Verification items for the finished model (mm, model axes). A direction names the side the tool comes from. Coordinates: 2 decimals unless noted, no trailing zeros. Loops run counter-clockwise (first coordinate to the right, second up) from the corner with the lowest first, then second, coordinate; pieces in that order, holes last. Notation, with made-up numbers: (-37, 73.5) - (13, 73.5) arc R28 cw to (13, 97.5) - close; hole circle Ø9 at (-19.5, -0.75). An arc over 180 degrees is marked (long way). One line per item, written item: value. Start each with the question number.
(1) Set-up check for faces 1 (the face through (-22.05, 5, 0)), 2 (the face through (-0.533, 3.491, 25.044)), 3 (the face through (15.799, 5.266, -11.984)): record each of +Z, -Z, +X, -X, +Y, -Y from which the full face is reachable in a straight line by a thin tool's end or side.
(2) Section check B-B (y = 3.25). Count the separate pieces of the cut face and the enclosed holes in it, plus the area to 3 significant figures.
(3) Gauge pin test, flat ends, axial feed: P1, Ø2, axis at y = 5.5, z = 0.5, coming from the +X side; P2, Ø0.8, axis at y = 3.5, z = 0.5, coming from the -X side; P3, Ø5, axis at x = 22, y = 5.5, coming from the +Z side; P4, Ø23.5, axis at x = 0, z = 0, coming from the -Y side. Record the tip position at first contact, or that the pin passes through.
(4) Draft check along Z on faces 4 (the face through (0.636, 10.258, -29.686)), 5 (the face through (24, 6, 1.25)), 6 (the face through (2, 6.4, 26)), 7 (the face through (7.91, 8.174, 10.316)). Enter one of: +Z half, -Z half, draft (parallel to the pull), parting line (faces both ways), or undercut.
(5) Thickness scan on probe 1 along X at (y, z) = (2, -0.5); probe 2 along Z at (x, y) = (18, 5.5); probe 3 along X at (y, z) = (6, 10). Record the ranges inside material, lowest first. Write a range as [from, to].
(6) Section check A-A (z = 0). Record the boundary of the cut face in (x, y) (3 decimals), plus the area to 3 significant figures.
```python
from build123d import *

# Parameters (mm, degrees)
SKETCH2_R               = 2.5
CUT_EXTRUDE1_DEPTH      = 44.751171413
SKETCH3_W               = 8
SKETCH3_H               = 2.5
CUT_EXTRUDE_THIN1_DEPTH = 44.751171413
CHAMFER1_SIZE           = 0.5


with BuildPart() as part:
    # Sketch1 → Revolve1 (revolve)
    with BuildSketch(Plane.XY, mode=Mode.PRIVATE) as revolve1_sk:
        Polygon((-15.975, 0), (-25.05, 0), (-25.05, 6.4), (-30.05, 6.4), (-30.05, 10.4), (-13, 10.4), (-13, 6.496321403), (-15.975, 4), align=None)
    revolve(revolve1_sk.sketch.rotate(Axis((0, 0, 0), (0, 1, 0)), 270), axis=Axis((0, 0, 0), (0, 1, 0)))

    # Sketch2 → Cut-Extrude1 (cut, through all)
    with BuildSketch(Plane(origin=(0, 10.4, 0), x_dir=(1, 0, 0), z_dir=(0, 1, 0))):
        with Locations(Location((0, 20, 0), (0, 0, 270))):
            Circle(SKETCH2_R)
        with Locations(Location((17.320508076, 10, 0), (0, 0, 270))):
            Circle(SKETCH2_R)
        with Locations(Location((17.320508076, -10, 0), (0, 0, 270))):
            Circle(SKETCH2_R)
        with Locations(Location((0, -20, 0), (0, 0, 270))):
            Circle(SKETCH2_R)
        with Locations(Location((-17.320508076, -10, 0), (0, 0, 270))):
            Circle(SKETCH2_R)
        with Locations(Location((-17.320508076, 10, 0), (0, 0, 270))):
            Circle(SKETCH2_R)
    extrude(amount=-CUT_EXTRUDE1_DEPTH, mode=Mode.SUBTRACT)

    # Sketch3 → Cut-Extrude-Thin1 (cut, through all)
    with BuildSketch(Plane(origin=(0, 10.4, 0), x_dir=(1, 0, 0), z_dir=(0, 1, 0))):
        with Locations((-26.05, 0)):
            Rectangle(SKETCH3_W, SKETCH3_H)
        with Locations((26.05, 0)):
            Rectangle(SKETCH3_W, SKETCH3_H)
    extrude(amount=-CUT_EXTRUDE_THIN1_DEPTH, mode=Mode.SUBTRACT)

    # Chamfer1
    chamfer1_edges = [part.edges().sort_by_distance(p)[0] for p in [
        (0, 0, 15.975),
        (0, 0, -22.5),
        (0, 10.4, -22.5),
        (-17.320508076, 0, -12.5),
        (-17.320508076, 10.4, -12.5),
        (-17.320508076, 0, 7.5),
        (-17.320508076, 10.4, 7.5),
        (0, 0, 17.5),
        (0, 10.4, 17.5),
        (17.320508076, 0, 7.5),
        (17.320508076, 10.4, 7.5),
        (17.320508076, 0, -12.5),
        (17.320508076, 10.4, -12.5),
        (0, 10.4, 30.05),
        (0, 10.4, -30.05),
        (26.036995204, 10.4, 1.25),
        (26.036995204, 10.4, -1.25),
        (-26.036995204, 10.4, -1.25),
        (-26.036995204, 10.4, 1.25),
        (0, 6.4, 30.05),
        (0, 6.4, -30.05),
        (0, 0, 25.05),
        (0, 0, -25.05),
        (-23.534396468, 0, -1.25),
        (-22.05, 0, 0),
        (-23.534396468, 0, 1.25),
        (-22.05, 10.4, 0),
        (0, 10.4, 13),
        (23.534396468, 0, 1.25),
        (22.05, 0, 0),
        (23.534396468, 0, -1.25),
        (22.05, 10.4, 0),
    ]]
    chamfer(chamfer1_edges, length=CHAMFER1_SIZE)


solid = part.part
```
Responses:
1. face 1: -X, +Y, -Y
1. face 2: +Z, -Y
1. face 3: +Y, -Y
2. separate pieces: 1
2. enclosed holes: 7
2. area: 1,040 mm²
3. P1: stops at x = 25.02
3. P2: stops at x = -22.05
3. P3: stops at z = 22.49
3. P4: passes through
4. face 4: -Z half
4. face 5: undercut
4. face 6: draft
4. face 7: undercut
5. probe 1: x = [-22.05, -15.97], [15.97, 22.05]
5. probe 2: z = [-17.42, -12.41], [-7.59, 7.59], [12.41, 17.42]
5. probe 3: x = [-22.97, -19.82], [-14.82, -9.2], [9.2, 14.82], [19.82, 22.97]
6. outline: (-22.05, 0.5) - (-21.55, 0) - (-16.475, 0) - (-15.975, 0.5) - (-15.975, 4) - (-13, 6.496) - (-13, 9.9) - (-13.5, 10.4) - (-21.55, 10.4) - (-22.05, 9.9) - close; (13, 6.496) - (15.975, 4) - (15.975, 0.5) - (16.475, 0) - (21.55, 0) - (22.05, 0.5) - (22.05, 9.9) - (21.55, 10.4) - (13.5, 10.4) - (13, 9.9) - close
6. area: 156 mm²
